Source: CAD feature listing. Evaluate the final solid. Frame: model axes, mm. Round coordinates to 2 decimals unless told otherwise and drop trailing zeros. Loops run counter-clockwise (first coordinate to the right, second up) from the corner with the lowest first, then second, coordinate; pieces in that order, holes last. Notation, with made-up numbers: M -15.75,10 L 39.25,10 A28 cw 39.25,37 Z; hole C 28,12 d5. An arc over 180 degrees is marked long. Answer as a JSON object with one key per item and string values.
Autodesk Inventor part; units mm, degrees
ref_plane "YZ Plane" through (0, 0, 0) normal (1, 0, 0) x (0, 1, 0)
ref_plane "XZ Plane" through (0, 0, 0) normal (0, 1, 0) x (-1, 0, 0)
ref_plane "XY Plane" through (0, 0, 0) normal (0, 0, 1) x (1, 0, 0)
sketch "Skizze1" plane through (0, 0, 0) normal (0, 0, 1) x (1, 0, 0)
  line L0 (0, 0) -> (0, 393.6564) construction
  line L1 (0, 0) -> (60, 0)
  line L2 (60, 0) -> (101.7513, 72.3153)
  line L3 (106.188, 80) -> (0, 80)
  arc A0 (106.6863, 76.0631) -> (101.7513, 72.3153) centre (108.6795, 68.3153) ccw
  arc A1 (106.6863, 76.0631) -> (106.188, 80) centre (106.188, 78) ccw
  line L4 (0, 0) -> (0, 80)
  dimension "d1" = 30
  dimension "d2" = 80
  dimension "d3" = 120
  dimension "d4" = 2
  dimension "d5" = 8
revolve "Umdrehung1" add sketch "Skizze1" angle 360 about axis through (0, 0, 0) along (0, 1, 0)
fillet "Rundung2" radius 35 1 edges at (-60, 0, 0)
shell "Wandung5" thickness 4 removed faces 2 at (6.6674, 80, -32.0854) at (-108.0747, 77.9307, -4.9241)
properties part number "Bol" material "Stahl, galvanisiert"
Item 1: Section C-C on z = 0. Return the cut outline in (x, y).
Answer sheet:
{"outline": "M -106.69,76.06 A8 cw -101.75,72.32 L -70.1,17.5 A35 ccw -39.79,0 L 39.79,0 A35 ccw 70.1,17.5 L 101.75,72.32 A8 cw 106.69,76.06 L 105.69,79.94 A12 ccw 98.29,74.32 L 66.64,19.5 A31 cw 39.79,4 L -39.79,4 A31 cw -66.64,19.5 L -98.29,74.32 A12 ccw -105.69,79.94 Z"}
Item 2: Pull-direction query (X, two-part tool) for faces 1 (the flat face through (-1, 0, -1)), 2 (the conical face through (-22.92, 79.69, -103.24)), 3 (the flat face through (-1, 4, -1)); classes: pulls with the +X half, pulls with the -X half, needs draft (parallel to the pull), parting line crosses it, or undercut.
Answer sheet:
{"face 1": "needs draft", "face 2": "parting line crosses it", "face 3": "undercut"}
Item 3: Section B-B on y = 50. Return the cut outline in (x, z).
Answer sheet:
{"outline": "C 0,0 d177.74; hole C 0,0 d168.5"}
Item 4: Contact query for flat-ended pins moving along their axis: pin 1 Ø24 at (x, z) = (20, 4.5) entering from +Y; pin 2 Ø12 at (x, z) = (19, 33.5) entering from +Y; pin 3 Ø8 at (x, y) = (-15.5, 42.5) entering from -Z. Output: stop coordinate, or through.
Answer sheet:
{"pin 1": "stops at y = 4", "pin 2": "stops at y = 4.36", "pin 3": "stops at z = -85.55"}
Item 5: Line query: probe 1 along X at (y, z) = (36, 11); probe 2 along Z at (x, y) = (35, 41.5); probe 3 along Z at (x, y) = (55, 50.5). Output: solid intervals per line, ascending. Write a range as from..to.
Answer sheet:
{"probe 1": "x = -80.03..-75.37, 75.37..80.03", "probe 2": "z = -76.32..-71.2, 71.2..76.32", "probe 3": "z = -70.17..-64.2, 64.2..70.17"}
Item 6: Section A-A on x = 0. Return the cut outline in (y, z), then the cut area to 3 significant figures.
Answer sheet:
{"outline": "M 0,-39.79 A35 ccw 17.5,-70.1 L 72.32,-101.75 A8 cw 76.06,-106.69 L 79.94,-105.69 A12 ccw 74.32,-98.29 L 19.5,-66.64 A31 cw 4,-39.79 L 4,39.79 A31 cw 19.5,66.64 L 74.32,98.29 A12 ccw 79.94,105.69 L 76.06,106.69 A8 cw 72.32,101.75 L 17.5,70.1 A35 ccw 0,39.79 Z", "area": "1,160 mm²"}
Item 7: Section D-D on y = 26. Return the cut outline in (x, z), then the cut area to 3 significant figures.
Answer sheet:
{"outline": "C 0,0 d150.02; hole C 0,0 d140.78", "area": "2,110 mm²"}
